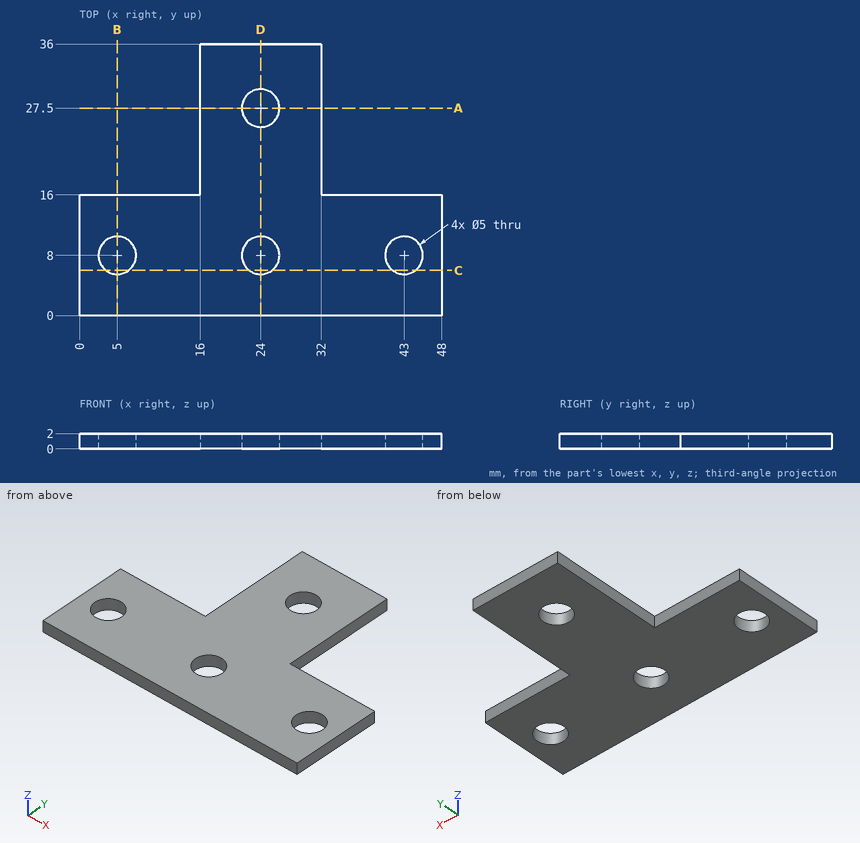
Verification items for this drawing (mm, ordinates from the low corner). Coordinates: 2 decimals unless noted, no trailing zeros. Write each loop counter-clockwise with the first axis right and the second up, starting at its lowest first coordinate (ties: lowest second). Pieces come first, ordered by that corner, then holes. Notation, with made-up numbers: (79, -24.75) -> (108, -24.75) arc R10 cw to (108, -20.75) -> close; hole circle Ø11 at (40.5, 70). An arc over 180 degrees is marked (long way). Use CSV: the item, a comma, the result in double quotes. Start each with the question number.
Item 1: Depth check by flat-ended pin: pin 1 Ø0.6 at (x, z) = (7.5, 1.5) entering from +Y; pin 2 Ø1 at (y, z) = (30.5, 1) entering from -X. Enter the tip coordinate at first touch or a pass-through.
Item 2: Cross-section at C-C, the plane y = 6. Record the cut outline in (x, z), plus the area to 3 significant figures.
Item 3: Thickness scan on line 1 (Y direction, x = 24, z = 0.7); line 2 (Y direction, x = 5, z = 1.25); line 3 (X direction, y = 31.5, z = 1.6). Record the ranges inside material, lowest first.
Item 4: Cross-section at B-B, the plane x = 5. Record the cut outline in (y, z), plus the area to 3 significant figures.
Item 5: Cross-section at D-D, the plane x = 24. Record the cut outline in (y, z), plus the area to 3 significant figures.
Item 6: Cross-section at A-A, the plane y = 27.5. Record the cut outline in (x, z).
Answers:
1,pin 1,"y = 16"
1,pin 2,"x = 16"
2,outline,"(0, 0) -> (3.5, 0) -> (3.5, 2) -> (0, 2) -> close; (6.5, 0) -> (22.5, 0) -> (22.5, 2) -> (6.5, 2) -> close; (25.5, 0) -> (41.5, 0) -> (41.5, 2) -> (25.5, 2) -> close; (44.5, 0) -> (48, 0) -> (48, 2) -> (44.5, 2) -> close"
2,area,"78.0 mm^2"
3,line 1,"0 to 5.5, 10.5 to 25, 30 to 36"
3,line 2,"0 to 5.5, 10.5 to 16"
3,line 3,"16 to 32"
4,outline,"(0, 0) -> (5.5, 0) -> (5.5, 2) -> (0, 2) -> close; (10.5, 0) -> (16, 0) -> (16, 2) -> (10.5, 2) -> close"
4,area,"22.0 mm^2"
5,outline,"(0, 0) -> (5.5, 0) -> (5.5, 2) -> (0, 2) -> close; (10.5, 0) -> (25, 0) -> (25, 2) -> (10.5, 2) -> close; (30, 0) -> (36, 0) -> (36, 2) -> (30, 2) -> close"
5,area,"52.0 mm^2"
6,outline,"(16, 0) -> (21.5, 0) -> (21.5, 2) -> (16, 2) -> close; (26.5, 0) -> (32, 0) -> (32, 2) -> (26.5, 2) -> close"
